Here's how the part is built. I have some questions about the finished solid (model axes, mm). A direction names the side the tool comes from. Coordinates: 2 decimals unless noted, no trailing zeros. Loops run counter-clockwise (first coordinate to the right, second up) from the corner with the lowest first, then second, coordinate; pieces in that order, holes last. Notation, with made-up numbers: (22, 73) - (28, 73) arc R18 cw to (28, 103) - close; hole circle Ø7 at (16.5, 60). An arc over 180 degrees is marked (long way). Use a Markdown table: item, result.
Autodesk Inventor part; units mm, degrees
ref_plane "Work Plane1" through (-43.1, -10, -10.1) normal (0, 0, -1) x (0, 1, 0)
ref_plane "Work Plane2" through (-43.1, -10, -10.1) normal (0, 0, -1) x (0, 1, 0)
ref_plane "YZ Plane" through (0, 0, 0) normal (1, 0, 0) x (0, 1, 0)
sketch "Sketch1" plane through (0, 0, 0) normal (0, 0, 1) x (1, 0, 0)
  circle A0 centre (0, 0) radius 3.1 construction
  line L0 (-5, 10) -> (-5, -10)
  line L1 (-5, -10) -> (19.1, -10) construction
  line L2 (19.1, -10) -> (19.1, 10)
  line L3 (19.1, 10) -> (-5, 10) construction
  line L4 (-33.5, -10) -> (-33.5, 10)
  line L5 (-33.5, 10) -> (-57.6, 10) construction
  line L6 (-57.6, -10) -> (-57.6, 10)
  line L7 (-57.6, -10) -> (-33.5, -10) construction
  circle A1 centre (-38.5, 0) radius 3.1 construction
  line L8 (-25.05, 5.3172) -> (-13.45, 5.3172)
  line L9 (19.1, -10.1) -> (-5, -10.1)
  line L10 (-5, -10.1) -> (-5, 1.6198)
  line L11 (-5, 10.1) -> (19.1, 10.1)
  line L12 (19.1, 10.1) -> (19.1, -10.1)
  line L13 (-33.5, -10.1) -> (-57.6, -10.1)
  line L14 (-57.6, -10.1) -> (-57.6, 10.1)
  line L15 (-57.6, 10.1) -> (-33.5, 10.1)
  line L16 (-33.5, 1.6198) -> (-33.5, -10.1)
  circle A2 centre (-38.5, 0) radius 3.2
  circle A3 centre (0, 0) radius 3
  arc A4 (-8.7654, 6.465) -> (-29.7346, 6.465) centre (-19.25, -34.6828) ccw
  line L17 (11.1, 18.1) -> (-49.6, 18.1)
  line L18 (-19.25, 5.3172) -> (-19.25, 9.0349) construction
  circle A5 centre (-16.25, 15.1) radius 1.65
  circle A6 centre (-22.25, 15.1) radius 1.65
  line L19 (11.1, 18.1) -> (19.1, 10.1)
  line L20 (-49.6, 18.1) -> (-57.6, 10.1)
  arc A7 (-29.7346, 6.465) -> (-33.5, 1.6198) centre (-28.5, 1.6198) ccw
  arc A8 (-5, 1.6198) -> (-8.7654, 6.465) centre (-10, 1.6198) ccw
  circle A9 centre (-19.25, 11.1) radius 1.65
  circle A10 centre (-19.25, 11.1) radius 1.65
  point P0 (0, 0)
  point P1 (-5, 5.3172)
  point P2 (-33.5, 5.3172)
  point P3 (-19.25, 18.1)
  point P4 (-5, 5.3172)
  point P5 (19.1, 10)
  point P6 (-33.5, 1.6198)
  point P7 (-5, 1.6198)
  dimension "d0" = 0.1
  dimension "d1" = 0.1
  dimension "d2" = 0.1
  dimension "d3" = 0.1
  dimension "d4" = 0.1
  dimension "d5" = 0.1
  dimension "d7" = 40
  dimension "d9" = 8
  dimension "d10" = 3
  dimension "d11" = 3.3
  dimension "d12" = 3
  dimension "d13" = 45
  dimension "d16" = 5
  dimension "d17" = 3.3
  dimension "d19" = 7
extrude "Extrusion1" add sketch "Sketch1" along normal blind 10
ref_plane "Work Plane1" through (-43.1, -10, -10.1) normal (0, 0, -1) x (0, 1, 0)
sketch "Sketch3" plane through (0, 0, 10) normal (0, 0, 1) x (1, 0, 0)
  line L0 (-33.5, -10.1) -> (-33.5, 1.6198)
  line L1 (-33.5, -10.1) -> (-57.6, -10.1)
  line L2 (-57.6, -10.1) -> (-57.6, -15.1)
  line L3 (-57.6, -15.1) -> (-33.5, -15.1)
  line L4 (-33.5, -15.1) -> (-33.5, -10.1)
  line L5 (-57.6, 10.1) -> (-57.6, -10.1)
  point P0 (0, 0)
  dimension "d25" = 5
extrude "Extrusion3" add sketch "Sketch3" against normal up to surface (20.1 mm away)
sketch "Sketch4" plane through (0, 0, 0) normal (0, 0, -1) x (-1, 0, 0)
  line L0 (33.5, -10) -> (33.5, 10) construction
  line L1 (33.5, 10) -> (57.6, 10) construction
  line L2 (57.6, -10) -> (57.6, 10) construction
  line L3 (57.6, -10) -> (33.5, -10) construction
  circle A0 centre (38.5, 0) radius 3.1 construction
  line L4 (-19.1, -10.1) -> (-19.1, 10.1) construction
  line L5 (5, -10.1) -> (-19.1, -10.1) construction
  line L6 (5, 1.6198) -> (5, -10.1) construction
  arc A1 (8.7654, 6.465) -> (5, 1.6198) centre (10, 1.6198) ccw construction
  arc A2 (29.7346, 6.465) -> (8.7654, 6.465) centre (19.25, -34.6828) ccw construction
  arc A3 (33.5, 1.6198) -> (29.7346, 6.465) centre (28.5, 1.6198) ccw construction
  line L7 (33.5, -10.1) -> (33.5, 1.6198) construction
  line L8 (57.6, -10.1) -> (33.5, -10.1) construction
  line L9 (57.6, 10.1) -> (57.6, -10.1) construction
  line L10 (49.6, 18.1) -> (57.6, 10.1)
  line L11 (-11.1, 18.1) -> (49.6, 18.1) construction
  line L12 (-19.1, 10.1) -> (-11.1, 18.1) construction
  circle A4 centre (19.25, 11.1) radius 1.65 construction
  circle A5 centre (16.25, 15.1) radius 1.65 construction
  circle A6 centre (0, 0) radius 3 construction
  circle A7 centre (38.5, 0) radius 3.2 construction
  circle A8 centre (22.25, 15.1) radius 1.65 construction
  line L13 (57.7, 10.1) -> (33.4, 10.1)
  line L14 (33.4, 10.1) -> (33.4, -10.1) construction
  line L15 (33.4, -10.1) -> (57.7, -10.1) construction
  line L16 (57.7, -10.1) -> (57.7, 10.1) construction
  line L17 (33.4, 10.1) -> (33.4, 18.1)
  line L18 (-11.1, 18.1) -> (49.6, 18.1)
  line L19 (49.6, 18.1) -> (57.6, 10.1)
  line L20 (33.4, 18.1) -> (49.6, 18.1)
  point P0 (0, 0)
  dimension "d28" = 0.1
ref_plane "Work Plane2" through (-43.1, -10, -10.1) normal (0, 0, -1) x (0, 1, 0)
extrude "Extrusion4" add sketch "Sketch4" along normal up to surface (10.1 mm away)
sketch "Sketch5" plane through (-49.6, 18.1, 10) normal (0, 1, 0) x (1, 0, 0)
  line L0 (16.1, 20.1) -> (16.1, 10.1) construction
  line L1 (-8, 10.1) -> (16.1, 10.1) construction
  line L2 (-8, 302.9) -> (-8, 10.1) construction
  line L3 (-8, 302.9) -> (68.7, 302.9) construction
  line L4 (68.7, 10.1) -> (68.7, 302.9) construction
  line L5 (44.6, 10.1) -> (68.7, 10.1) construction
  line L6 (44.6, 10.1) -> (44.6, 20.1) construction
  line L7 (44.6, 20.1) -> (54.2, 20.1) construction
  arc A0 (54.2, 20.1) -> (59.2, 25.1) centre (54.2, 25.1) ccw construction
  line L8 (59.2, 175.1) -> (59.2, 25.1) construction
  arc A1 (59.2, 175.1) -> (54.2, 180.1) centre (54.2, 175.1) ccw construction
  line L9 (6.5, 180.1) -> (54.2, 180.1) construction
  arc A2 (6.5, 180.1) -> (1.5, 175.1) centre (6.5, 175.1) ccw construction
  line L10 (1.5, 25.1) -> (1.5, 175.1) construction
  arc A3 (1.5, 25.1) -> (6.5, 20.1) centre (6.5, 25.1) ccw construction
  line L11 (16.1, 20.1) -> (6.5, 20.1) construction
  circle A4 centre (63.7, 292.9) radius 2.15 construction
  circle A5 centre (-3, 273) radius 2.15 construction
  circle A6 centre (-3, 292.9) radius 2.15 construction
  circle A7 centre (63.7, 273) radius 2.15 construction
  circle A8 centre (10.85, 15.1) radius 2.5 construction
  circle A9 centre (49.85, 15.1) radius 2.5 construction
  line L12 (-8, 10) -> (-8, 20.1)
  line L13 (16.2, 10) -> (16.2, 20.1)
  line L14 (-8, 10) -> (16.2, 10)
  line L15 (16.2, 10) -> (16.2, 20.1)
  line L16 (16.2, 20.1) -> (-8, 20.1)
  line L17 (-8, 20.1) -> (-8, 10)
  point P0 (49.6, 10)
extrude "Extrusion5" cut sketch "Sketch5" against normal blind 3
sketch "Sketch6" plane through (-49.6, 15.1, 10) normal (0, 1, 0) x (1, 0, 0)
  circle A0 centre (10.85, 15.1) radius 2.5 construction
  circle A1 centre (10.85, 15.1) radius 2.8
  point P0 (49.6, 10)
  dimension "d33" = 0.3
extrude "Extrusion6" cut sketch "Sketch6" against normal through all
fillet "Fillet2" radius 1 1 edges at (-43, 15.1, 0)
ref_plane "Work Plane3" through (-19.25, -15.1, 10) normal (-1, 0, 0) x (0, 0, 1)
mirror "Mirror1" about plane through (-19.25, -15.1, 10) normal (-1, 0, 0) of "Extrusion3", "Extrusion4", "Extrusion5", "Extrusion6", "Fillet2"
ref_plane "Work Plane4" through (4.6, -10, -10.1) normal (0, 0, 1) x (0, 1, 0)
equation "\"d17\" = d11"
properties part number "pivot module base"
Q1. I want a section at A-A, the plane z = -5.1. Give the number of separate pieces and of enclosed holes in the cut face, then the cut area to 3 significant figures.
Check values:
| item | result |
|---|---|
| separate pieces | 8 |
| enclosed holes | 0 |
| area | 346 mm^2 |
Q2. Which directions (+Z, -Z, +X, -X, +Y, -Y) give clear straight access to the entire face, cutting with the end or side of a thin tool? Please do faces 1 (the face through (-46, -13, -10.1)), 2 (the face through (4, 15.1, -6)), 3 (the face through (-6.081, 4.724, 4.93)), 4 (the face through (7, -10.1, -5)).
Check values:
| item | result |
|---|---|
| face 1 | -Z, +X, -X, +Y, -Y |
| face 2 | -Z, +X, -X, +Y |
| face 3 | +Z, -Z, -Y |
| face 4 | -Z, +X, -X |
Q3. If we mould it in two halves opening along Z, with no side actions, what happens to faces 5 (the face through (0.857, 12.635, -7.833)), 6 (the face through (-43, 15.1, -6)), 7 (the face through (7, 13, -10.1))? For each: pulls with the +Z half, pulls with the -Z half, needs draft (parallel to the pull), parting line crosses it, or undercut.
Check values:
| item | result |
|---|---|
| face 5 | undercut |
| face 6 | needs draft |
| face 7 | pulls with the -Z half |
Q4. I want a section at B-B, the plane y = 11.1. Write out the boundary of the cut face in (x, z).
Check values:
| item | result |
|---|---|
| outline | (-56.6, -10.1) - (-33.4, -10.1) - (-33.4, 0) - (-20.9, 0) - (-20.9, 10) - (-56.6, 10) - close; (-17.6, 0) - (-5.1, 0) - (-5.1, -10.1) - (18.1, -10.1) - (18.1, 10) - (-17.6, 10) - close; hole circle Ø5.6 at (-38.75, -5.1); hole circle Ø5.6 at (0.25, -5.1) |
Q5. I want a section at D-D, the plane x = -19.25. Write out the boundary of the cut face in (y, z), then the cut area to 3 significant figures.
Check values:
| item | result |
|---|---|
| outline | (7.78, 0) - (9.45, 0) - (9.45, 10) - (7.78, 10) - close; (12.75, 0) - (18.1, 0) - (18.1, 10) - (12.75, 10) - close |
| area | 70.2 mm^2 |
Q6. Will these pins go through, and if not, where does the flat tip stop? P1, Ø10, axis at x = -26.5, z = 6.5, coming from the -Y side; P2, Ø5, axis at x = -38.75, z = -5.1, coming from the +Y side; P3, Ø5, axis at y = 12, z = -2.5, coming from the +X side; P4, Ø3, axis at x = 7.5, z = -6.5, coming from the +Y side.
Check values:
| item | result |
|---|---|
| P1 | y = 5.62 |
| P2 | through |
| P3 | x = 19.1 |
| P4 | y = 15.1 |
Q7. I want a section at C-C, the plane y = -4. Write out the boundary of the cut face in (x, z).
Check values:
| item | result |
|---|---|
| outline | (-57.6, 0) - (-33.5, 0) - (-33.5, 10) - (-57.6, 10) - close; (-5, 0) - (19.1, 0) - (19.1, 10) - (-5, 10) - close |
Q8. Please list where these lines run through material, in increasing order: L1, parallel to Z at x = 0, y = -13; L2, parallel to Y at x = -41, z = -3.25; L3, parallel to Z at x = 13.5, y = -6.5. Write a range as from..to.
Check values:
| item | result |
|---|---|
| L1 | -10.1..-7.89, -2.31..10 |
| L2 | -15.1..-10.1, 10.1..15.1 |
| L3 | 0..10 |
